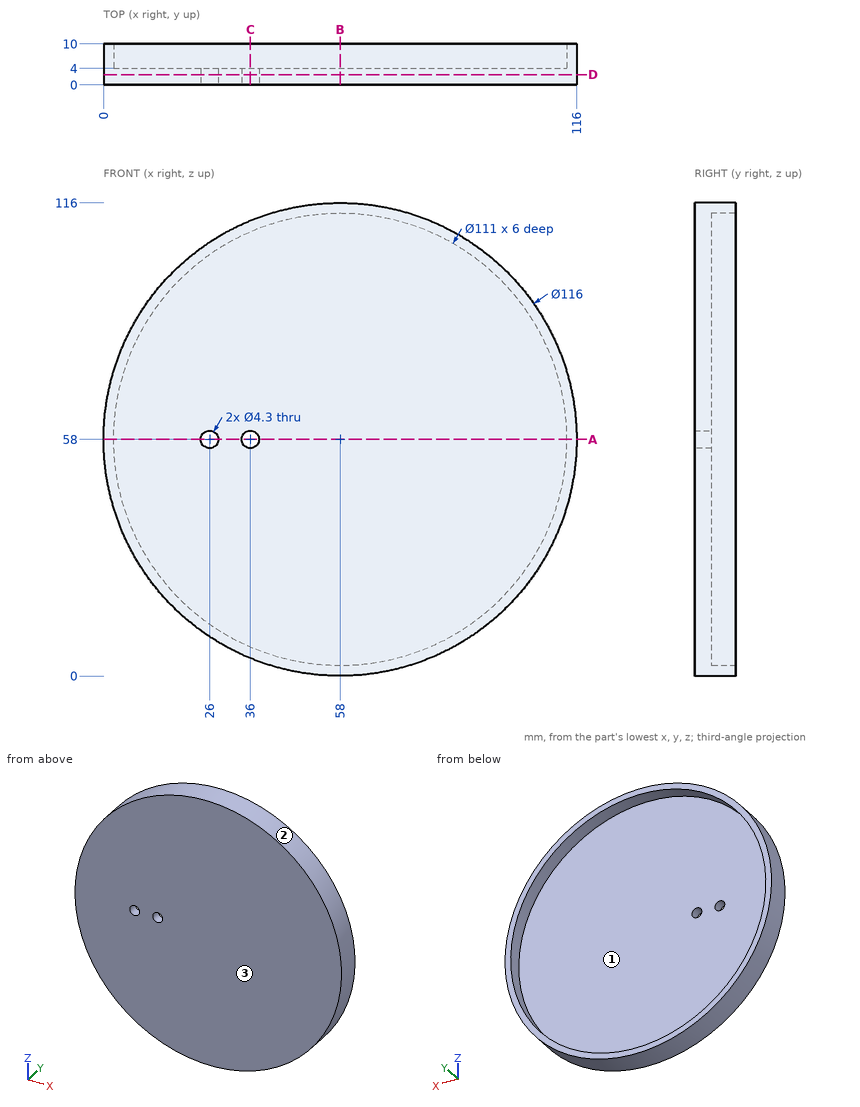
Geometry check sheet. Reference: drawing and pictorial views, mm from the part's lowest x, y, z. Coordinates: 2 decimals unless noted, no trailing zeros. Order: outer loops, then holes, each group sorted by start corner. A loop starts at its lowest first (then second) coordinate and runs counter-clockwise, first axis right, second up. Notation, with made-up numbers: M 50,53.25 L 103,53.25 A21 ccw 103,75.25 Z; hole C 51.5,17 d10. An arc over 180 degrees is marked long. Return JSON: item names as keys, results as strings.
1) Thickness scan on L1, parallel to X at y = 1.55, z = 58; L2, parallel to X at y = 5.75, z = 58; L3, parallel to Y at x = 24.5, z = 63.5. Record the ranges inside material, lowest first. Write a range as [from, to].
Answer list:
{"L1": "[0, 23.85], [28.15, 33.85], [38.15, 116]", "L2": "[0, 2.5], [113.5, 116]", "L3": "[0, 4]"}
2) Cross-section at D-D, the plane y = 2.5. Record the boundary of the cut face in (x, z).
Answer list:
{"outline": "C 58,58 d116; hole C 26,58 d4.3; hole C 36,58 d4.3"}
3) Cross-section at B-B, the plane x = 58. Record the boundary of the cut face in (y, z), and give its area (3 significant figures).
Answer list:
{"outline": "M 0,0 L 10,0 L 10,2.5 L 4,2.5 L 4,113.5 L 10,113.5 L 10,116 L 0,116 Z", "area": "494 mm2"}
4) Cross-section at A-A, the plane z = 58. Record the boundary of the cut face in (x, y), and give its area (3 significant figures).
Answer list:
{"outline": "M 0,0 L 23.85,0 L 23.85,4 L 2.5,4 L 2.5,10 L 0,10 Z; M 28.15,0 L 33.85,0 L 33.85,4 L 28.15,4 Z; M 38.15,0 L 116,0 L 116,10 L 113.5,10 L 113.5,4 L 38.15,4 Z", "area": "460 mm2"}
5) Cross-section at C-C, the plane x = 36. Record the boundary of the cut face in (y, z).
Answer list:
{"outline": "M 0,4.33 L 10,4.33 L 10,7.05 L 4,7.05 L 4,55.85 L 0,55.85 Z; M 0,60.15 L 4,60.15 L 4,108.95 L 10,108.95 L 10,111.67 L 0,111.67 Z"}
6) Release check for a two-part mould opening along X. For the marked faces 1, 2 and 3 record: +X half, -X half, draft (parallel to the pull), parting line (faces both ways), or undercut.
Answer list:
{"face 1": "undercut", "face 2": "parting line", "face 3": "draft"}
7) Gauge pin test, flat ends, axial feed: pin 1 (4 mm diameter, centred on x = 36, z = 58, fed in from +Y); pin 2 (4 mm diameter, centred on y = 6.5, z = 44.5, fed in from +X); pin 3 (3 mm diameter, centred on x = 51.5, y = 2, fed in from +Z); pin 4 (1 mm diameter, centred on y = 4, z = 45.5, fed in from +X). Record the tip position at first contact, or that the pin passes through.
Answer list:
{"pin 1": "through", "pin 2": "x = 114.85", "pin 3": "z = 115.78", "pin 4": "x = 114.75"}
